```python
from build123d import *

# Parameters (mm, degrees)
BOSS_EXTRUDE1_DEPTH = 2
SKETCH2_W           = 11
SKETCH2_H           = 8
BOSS_EXTRUDE2_DEPTH = 7
SKETCH3_R           = 2
CUT_EXTRUDE2_DEPTH  = 83.38476801
BOSS_EXTRUDE3_DEPTH = 2
SHELL1_START        = 0.25
SHELL1_DEPTH        = 3.75
SHELL1_2_OUTLINE_R  = 2.25
SHELL1_2_DEPTH      = 1.5
SHELL1_START_2      = -6.75
SHELL1_3_OUTLINE_W  = 10.5
SHELL1_3_OUTLINE_H  = 7.5
SHELL1_3_OUTLINE_R  = 2.25
SHELL1_3_DEPTH      = 7
RIB2_REACH          = 84.627
BOSS_EXTRUDE4_DEPTH = 2


# Read off the part's stored shape, not the designer's step: Shell1
with BuildPart() as part:
    # Sketch1 → Boss-Extrude1 (new body)
    with BuildSketch(Plane(origin=(0, 0, 0), x_dir=(1, 0, 0), z_dir=(0, 1, 0))):
        with BuildLine():
            Line((0, 0), (0, 17.5))
            Line((0, 17.5), (41.207252266, 10.607357821))
            ThreePointArc((41.207252266, 10.607357821), (51.063628859, 9.311158863), (61, 9))
            Line((61, 9), (80, 9))
            Line((80, 9), (80, 0))
            Line((80, 0), (0, 0))
        make_face()
    extrude(amount=BOSS_EXTRUDE1_DEPTH)

    # Sketch2 → Boss-Extrude2 (add)
    with BuildSketch(Plane.XZ):
        with Locations((49.982902032, -4)):
            Rectangle(SKETCH2_W, SKETCH2_H)
    extrude(amount=BOSS_EXTRUDE2_DEPTH)

    # Sketch3 → Cut-Extrude2 (cut, through all)
    with BuildSketch(Plane.XZ.offset(7)):
        with Locations(Location((49.982902032, -4, 0), (0, 0, 270))):
            Circle(SKETCH3_R)
    extrude(amount=-CUT_EXTRUDE2_DEPTH, mode=Mode.SUBTRACT)

    # Sketch4 → Boss-Extrude3 (add)
    with BuildSketch(Plane(origin=(0, 2, 0), x_dir=(1, 0, 0), z_dir=(0, 1, 0))):
        Polygon((40.877300801, 8.634762569), (41, 2), (2, 2), (2, 15.137679132), align=None)
    extrude(amount=BOSS_EXTRUDE3_DEPTH)

    # Shell1 outline → Shell1 (cut)
    with BuildSketch(Plane(origin=(0, 0, 0), x_dir=(1, 0, 0), z_dir=(0, 1, 0)).offset(SHELL1_START)):
        Polygon((2.25, 2.25), (40.745333907, 2.25), (40.631184307, 8.422456723), (2.25, 14.842389024), align=None)
    extrude(amount=SHELL1_DEPTH, mode=Mode.SUBTRACT)

    # Shell1 2 outline → Shell1 2 (cut)
    with BuildSketch(Plane(origin=(0, 0, 0), x_dir=(1, 0, 0), z_dir=(0, 1, 0)).offset(SHELL1_START)):
        with BuildLine():
            Line((79.75, 0.25), (79.75, 8.75))
            Line((79.75, 8.75), (61.002301351, 8.75))
            ThreePointArc((61.002301351, 8.75), (51.043164326, 9.06199776), (41.164190751, 10.361087437))
            Line((41.164190751, 10.361087437), (0.25, 17.204709892))
            Line((0.25, 17.204709892), (0.25, 0.25))
            Line((0.25, 0.25), (79.75, 0.25))
        make_face()
        Polygon((40.631184307, 8.422456723), (40.745333907, 2.25), (2.25, 2.25), (2.25, 14.842389024), align=None, mode=Mode.SUBTRACT)
        with Locations((49.982902032, 4)):
            Circle(SHELL1_2_OUTLINE_R, mode=Mode.SUBTRACT)
    extrude(amount=SHELL1_2_DEPTH, mode=Mode.SUBTRACT)

    # Shell1 3 outline → Shell1 3 (cut)
    with BuildSketch(Plane(origin=(0, 0, 0), x_dir=(1, 0, 0), z_dir=(0, 1, 0)).offset(SHELL1_START_2)):
        with Locations((49.982902032, 4)):
            Rectangle(SHELL1_3_OUTLINE_W, SHELL1_3_OUTLINE_H)
        with Locations((49.982902032, 4)):
            Circle(SHELL1_3_OUTLINE_R, mode=Mode.SUBTRACT)
    extrude(amount=SHELL1_3_DEPTH, mode=Mode.SUBTRACT)

    # Sketch8 walls → Rib2 (add, up to next)
    with BuildSketch(Plane(origin=(0, 4, 0), x_dir=(1, 0, 0), z_dir=(0, 1, 0)), mode=Mode.PRIVATE) as rib2_sk1:
        Polygon((-30.5404545, 90.126090222), (45.840432464, -73.587738012), (46.06698827, -73.482038123), (-30.313898694, 90.231790111), align=None)
    rib2_tool1 = extrude(rib2_sk1.sketch, amount=-RIB2_REACH, mode=Mode.PRIVATE) - part.part
    # Sketch8 walls → Rib2 (add, up to next)
    with BuildSketch(Plane(origin=(0, 4, 0), x_dir=(1, 0, 0), z_dir=(0, 1, 0)), mode=Mode.PRIVATE) as rib2_sk2:
        Polygon((48.244103521, 88.119990894), (-32.940634825, -72.310767507), (-32.717569751, -72.423647853), (48.467168595, 88.007110547), align=None)
    rib2_tool2 = extrude(rib2_sk2.sketch, amount=-RIB2_REACH, mode=Mode.PRIVATE) - part.part
    # Sketch8 walls → Rib2 (add, up to next)
    with BuildSketch(Plane(origin=(0, 4, 0), x_dir=(1, 0, 0), z_dir=(0, 1, 0)), mode=Mode.PRIVATE) as rib2_sk3:
        Polygon((-19.945501862, 88.559114212), (54.930872718, -73.737760739), (55.15787846, -73.633030645), (-19.718496119, 88.663844307), align=None)
    rib2_tool3 = extrude(rib2_sk3.sketch, amount=-RIB2_REACH, mode=Mode.PRIVATE) - part.part
    # Sketch8 walls → Rib2 (add, up to next)
    with BuildSketch(Plane(origin=(0, 4, 0), x_dir=(1, 0, 0), z_dir=(0, 1, 0)), mode=Mode.PRIVATE) as rib2_sk4:
        Polygon((57.294710169, 86.727791097), (-22.305946259, -72.494493497), (-22.082333571, -72.606285115), (57.518322857, 86.615999479), align=None)
    rib2_tool4 = extrude(rib2_sk4.sketch, amount=-RIB2_REACH, mode=Mode.PRIVATE) - part.part
    # Sketch8 walls → Rib2 (add, up to next)
    with BuildSketch(Plane(origin=(0, 4, 0), x_dir=(1, 0, 0), z_dir=(0, 1, 0)), mode=Mode.PRIVATE) as rib2_sk5:
        Polygon((-21.175633704, 75.686160498), (88.535096121, -63.505624935), (88.731438538, -63.350868173), (-20.979291286, 75.840917259), align=None)
    rib2_tool5 = extrude(rib2_sk5.sketch, amount=-RIB2_REACH, mode=Mode.PRIVATE) - part.part
    # Sketch8 walls → Rib2 (add, up to next)
    with BuildSketch(Plane(origin=(0, 4, 0), x_dir=(1, 0, 0), z_dir=(0, 1, 0)), mode=Mode.PRIVATE) as rib2_sk6:
        Polygon((92.986420538, 71.052239579), (-25.615710829, -59.5819061), (-25.430615704, -59.749953101), (93.171515663, 70.884192578), align=None)
    rib2_tool6 = extrude(rib2_sk6.sketch, amount=-RIB2_REACH, mode=Mode.PRIVATE) - part.part
    add(rib2_tool1.solids().sort_by_distance((7.763266885, 4, -8.32202605))[0])
    add(rib2_tool2.solids().sort_by_distance((7.763266885, 4, -7.84817152))[0])
    add(rib2_tool3.solids().sort_by_distance((17.606188299, 4, -7.463041784))[0])
    add(rib2_tool4.solids().sort_by_distance((17.606188299, 4, -7.060752991))[0])
    add(rib2_tool5.solids().sort_by_distance((33.777902417, 4, -6.167646162))[0])
    add(rib2_tool6.solids().sort_by_distance((33.777902417, 4, -5.651143239))[0])

    # Sketch9 → Boss-Extrude4 (add)
    with BuildSketch(Plane(origin=(0, 2, 0), x_dir=(1, 0, 0), z_dir=(0, 1, 0))):
        Polygon((77.681321794, 6.50188709), (77.681321794, 2.50188709), (57.121277642, 1), (57.121277642, 8.00377418), align=None)
    extrude(amount=BOSS_EXTRUDE4_DEPTH)


solid = part.part
```
The listing builds one solid part. Answer for the finished solid, in the listing's coordinates (mm). A direction names the side the tool comes from. Give positions to 0.01 mm unless a question says otherwise; leave off trailing zeros. Order: outer loops, then holes, each group sorted by start corner. A loop starts at its lowest first (then second) coordinate and runs counter-clockwise, first axis right, second up.
Item 1: The part is cut by section B-B, the plane x = 66. Give the vertices of the cut face in (y, z).
From the geometry:
outline: (0, -9) - (2, -9) - (2, -7.36) - (4, -7.36) - (4, -1.65) - (2, -1.65) - (2, 0) - (0, 0) - close; hole (0.25, -8.75) - (1.75, -8.75) - (1.75, -0.25) - (0.25, -0.25) - close
Item 2: The part is cut by section C-C, the plane z = -4. Count the separate pieces of the cut face and the enclosed holes in it, and give its area (3 significant figures).
From the geometry:
separate pieces: 2
enclosed holes: 1
area: 85.6 mm2
Item 3: The part is cut by section D-D, the plane x = 9. Give the vertices of the cut face in (y, z).
From the geometry:
outline: (0, -15.99) - (2, -15.99) - (2, -13.97) - (4, -13.97) - (4, -13.71) - (1.75, -13.71) - (1.75, -15.74) - (0.25, -15.74) - (0.25, -10.57) - (4, -10.57) - (4, -10.02) - (0.25, -10.02) - (0.25, -5.97) - (4, -5.97) - (4, -5.38) - (0.25, -5.38) - (0.25, -0.25) - (1.75, -0.25) - (1.75, -2.25) - (4, -2.25) - (4, -2) - (2, -2) - (2, 0) - (0, 0) - close
Item 4: Which of the six approach directions +Z, -Z, +X, -X, +Y, -Y give full straight-line access (tool end or side, diameter ignored) to faces 3 (the face through (25, 3, -2.25)), 4 (the face through (13, 0.25, -8)), 5 (the face through (50, -3, -8)), 6 (the face through (2, 3, -8)), 7 (the face through (70, 1, -9))?
From the geometry:
face 3: +Y
face 4: none
face 5: -Z, +X, -X, -Y
face 6: +Z, -Z, -X, +Y
face 7: -Z, +X, +Y, -Y
Item 5: For a pull along Y with two mould halves and no side action, classify faces 1 (the face through (34, 3, -2.25)), 2 (the face through (18, 0.25, -2)) as pulls with the +Y half, pulls with the -Y half, needs draft (parallel to the pull), parting line crosses it, or undercut.
From the geometry:
face 1: needs draft
face 2: undercut
Item 6: Find the intervals of material crossed by probe 1 along X at (y, z) = (-1.5, -4); probe 2 along Y at (x, z) = (35.5, -9.75); probe 3 along X at (y, z) = (-5.75, -5.75), in increasing order.
From the geometry:
probe 1: x = 44.48 to 44.73, 47.73 to 47.98, 51.98 to 52.23, 55.23 to 55.48
probe 2: y = 0 to 0.25, 1.75 to 2
probe 3: x = 44.48 to 44.73, 48.57 to 49.01, 50.95 to 51.4, 55.23 to 55.48
Item 7: Given pin 1 Ø0.7 at (x, y) = (8.5, 2.5) entering from -Z; pin 2 Ø1.6 at (x, y) = (2, 1) entering from -Z; pin 3 Ø2 at (x, z) = (62.5, -2.5) entering from -Y; pin 4 Ø5 at (x, y) = (67.5, -0.5) entering from +Z, each flat-ended and moving along its own axis, determine where each tip first touches the part or whether it passes through.
From the geometry:
pin 1: stops at z = -14.11
pin 2: stops at z = -17.3
pin 3: stops at y = 0
pin 4: stops at z = 0
Item 8: The part is cut by section A-A, the plane y = -5.5. Give the vertices of the cut face in (x, z), and give its area (3 significant figures).
From the geometry:
outline: (44.48, -8) - (55.48, -8) - (55.48, 0) - (44.48, 0) - close; circle Ø4.5 at (49.98, -4); hole (44.73, -7.75) - (55.23, -7.75) - (55.23, -0.25) - (44.73, -0.25) - close; hole circle Ø4 at (49.98, -4)
area: 12.6 mm2
